Build history of the part. All positions in model axes, mm. A direction names the side the tool comes from. Round coordinates to 2 decimals unless told otherwise and drop trailing zeros. Write each loop counter-clockwise with the first axis right and the second up, starting at its lowest first coordinate (ties: lowest second). Pieces come first, ordered by that corner, then holes. Notation, with made-up numbers: (81, 60.5) - (107, 60.5) arc R14 cw to (107, 72.5) - close; hole circle Ø1 at (-19.5, 0.5). An arc over 180 degrees is marked (long way). Answer as a JSON object with one key per item and string values. Group by question number.
Item 1: Probe line 1 (Z direction, x = 81, y = 137); line 2 (X direction, y = 45, z = 129). List the from-to ranges inside material, lowest first. Write a range as from..to.
Item 2: Slice it at A-A, the plane y = 144. List the corners of the cut face in (x, z).
Item 3: Which spindle directions (+Z, -Z, +X, -X, +Y, -Y) get a long thin tool onto all of the face, cutting with end or side? Do faces 4 (the cylindrical face through (-4.17, 111.71, 126.82)), 5 (the flat face through (-1, 80, -114.3)). Say none if no direction does.
Item 4: Two-plate mould, pull along Y, no slides. Class faces 1 (the cylindrical face through (-58.953, 21.536, 126.822)), 2 (the flat face through (88.9, 80, 2)), 3 (the flat face through (-1, 0, -2)): +Y half, -Y half, draft (parallel to the pull), parting line (faces both ways), or undercut.
Item 5: Flat gauge pin, fed straight in: pin 1 (12 mm diameter, centred on x = 8, y = 125, fed in from +Z). Where does the tip first touch, or does it go through?
from build123d import *

# Parameters (mm, degrees)
SKETCH1_W           = 177.8
SKETCH1_H           = 228.6
BOSS_EXTRUDE1_DEPTH = 161.925
SKETCH2_R           = 6.35
BOSS_EXTRUDE2_DEPTH = 25.4
SKETCH4_R           = 6.35
BOSS_EXTRUDE4_DEPTH = 25.4
LPATTERN1_COUNT     = 2
LPATTERN1_PITCH     = 25.4
LPATTERN2_COUNT     = 2
LPATTERN2_PITCH     = 25.4
SKETCH5_R           = 1.27
BOSS_EXTRUDE5_DEPTH = 12.7
LPATTERN3_COUNT     = 2
LPATTERN3_PITCH     = 25.4
SKETCH6_R           = 1.27
BOSS_EXTRUDE6_DEPTH = 12.7
LPATTERN4_COUNT     = 2
LPATTERN4_PITCH     = 25.4


with BuildPart() as part:
    # Sketch1 → Boss-Extrude1 (new body)
    with BuildSketch(Plane(origin=(0, 0, 0), x_dir=(1, 0, 0), z_dir=(0, 1, 0))):
        Rectangle(SKETCH1_W, SKETCH1_H)
    extrude(amount=BOSS_EXTRUDE1_DEPTH)

    # Sketch2 → Boss-Extrude2 (add)
    with BuildSketch(Plane.XY.offset(114.3)):
        with Locations((-2.792336917, 117.907265363)):
            Circle(SKETCH2_R)
    boss_extrude2 = extrude(amount=BOSS_EXTRUDE2_DEPTH)

    # Sketch4 → Boss-Extrude4 (add)
    with BuildSketch(Plane.XY.offset(114.3)):
        with Locations((-53.913582013, 25.4)):
            Circle(SKETCH4_R)
    boss_extrude4 = extrude(amount=BOSS_EXTRUDE4_DEPTH)

    # LPattern1: Boss-Extrude2 ×2
    with Locations(*[(0, -i * LPATTERN1_PITCH, 0) for i in range(1, LPATTERN1_COUNT)]):
        add(boss_extrude2)

    # LPattern2: Boss-Extrude4 ×2
    with Locations(*[(0, i * LPATTERN2_PITCH, 0) for i in range(1, LPATTERN2_COUNT)]):
        add(boss_extrude4)

    # Sketch5 → Boss-Extrude5 (add)
    with BuildSketch(Plane.XY.offset(139.7)):
        with Locations((-2.730512125, 118.079738131)):
            Circle(SKETCH5_R)
    boss_extrude5 = extrude(amount=BOSS_EXTRUDE5_DEPTH)

    # LPattern3: Boss-Extrude5 ×2
    with Locations(*[(0, -i * LPATTERN3_PITCH, 0) for i in range(1, LPATTERN3_COUNT)]):
        add(boss_extrude5)

    # Sketch6 → Boss-Extrude6 (add)
    with BuildSketch(Plane.XY.offset(139.7)):
        with Locations((-53.913582013, 50.8)):
            Circle(SKETCH6_R)
    boss_extrude6 = extrude(amount=BOSS_EXTRUDE6_DEPTH)

    # LPattern4: Boss-Extrude6 ×2
    with Locations(*[(0, -i * LPATTERN4_PITCH, 0) for i in range(1, LPATTERN4_COUNT)]):
        add(boss_extrude6)


solid = part.part
Geometry says:
{
 "1": {"line 1": "z = -114.3..114.3", "line 2": "x = -56.5..-51.33"},
 "2": {"outline": "(-88.9, -114.3) - (88.9, -114.3) - (88.9, 114.3) - (-88.9, 114.3) - close"},
 "3": {"face 4": "+Z", "face 5": "-Z, +X, -X, +Y, -Y"},
 "4": {"face 1": "undercut", "face 2": "draft", "face 3": "-Y half"},
 "5": {"pin 1": "stops at z = 114.3"}
}
